Could you check a few things on this model? Use its own coordinates, in mm. Face numbers are marked on the shaded views. A direction names the side the tool comes from. Give positions to 0.01 mm unless a question says otherwise; leave off trailing zeros. Write each loop counter-clockwise with the first axis right and the second up, starting at its lowest first coordinate (ties: lowest second). Pieces come first, ordered by that corner, then holes. Notation, with made-up numbers: (-29.75, -30.5) - (-17.75, -30.5) arc R13 cw to (-17.75, -16.5) - close; hole circle Ø5 at (-21, -9). An arc over 180 degrees is marked (long way). Write item = value, one per line.
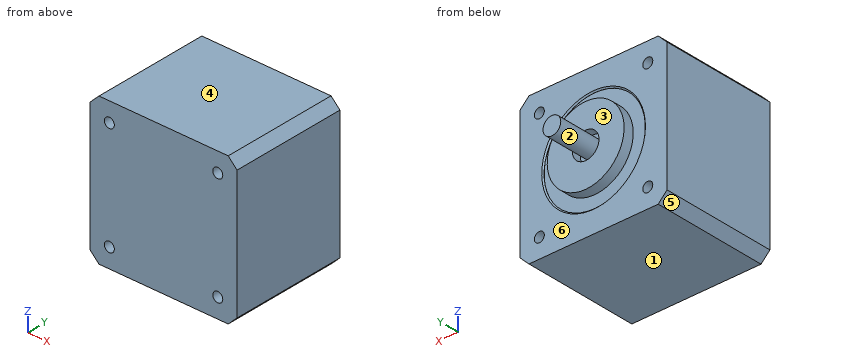
from build123d import *

# Parameters (mm, degrees)
SKETCH1_W           = 42.037
SKETCH1_H           = 42.037
BOSS_EXTRUDE1_DEPTH = 33.02
CHAMFER1_SIZE       = 2.54
SKETCH2_R           = 10.9982
SKETCH2_R_2         = 3.81
BOSS_EXTRUDE2_DEPTH = 2.54
CUT_EXTRUDE1_START  = -0.381
SKETCH3_R           = 14.478
SKETCH3_R_2         = 10.9982
CUT_EXTRUDE1_DEPTH  = 0.381
CHAMFER2_SIZE       = 0.3556
SKETCH4_R           = 2.54
BOSS_EXTRUDE3_DEPTH = 13.3858
SKETCH5_R           = 1.4224
CUT_EXTRUDE2_DEPTH  = 45.428313996


with BuildPart() as part:
    # Sketch1 → Boss-Extrude1 (new body)
    with BuildSketch(Plane(origin=(0, 0, 0), x_dir=(1, 0, 0), z_dir=(0, 1, 0))):
        Rectangle(SKETCH1_W, SKETCH1_H)
    extrude(amount=BOSS_EXTRUDE1_DEPTH)

    # Chamfer1
    chamfer1_edges = [part.edges().sort_by_distance(p)[0] for p in [
        (21.0185, 16.51, 21.0185),
        (-21.0185, 16.51, 21.0185),
        (-21.0185, 16.51, -21.0185),
        (21.0185, 16.51, -21.0185),
    ]]
    chamfer(chamfer1_edges, length=CHAMFER1_SIZE)

    # Sketch2 → Boss-Extrude2 (add)
    with BuildSketch(Plane(origin=(0, 33.02, 0), x_dir=(1, 0, 0), z_dir=(0, 1, 0))):
        with Locations(Location((0, 0, 0), (0, 0, 90))):
            Circle(SKETCH2_R)
        with Locations(Location((0, 0, 0), (0, 0, 270))):
            Circle(SKETCH2_R_2, mode=Mode.SUBTRACT)
    extrude(amount=BOSS_EXTRUDE2_DEPTH)

    # Sketch3 → Cut-Extrude1 (cut)
    with BuildSketch(Plane(origin=(0, 33.02, 0), x_dir=(1, 0, 0), z_dir=(0, 1, 0)).offset(CUT_EXTRUDE1_START)):
        with Locations(Location((0, 0, 0), (0, 0, 270))):
            Circle(SKETCH3_R)
        with Locations(Location((0, 0, 0), (0, 0, 270))):
            Circle(SKETCH3_R_2, mode=Mode.SUBTRACT)
    extrude(amount=CUT_EXTRUDE1_DEPTH, mode=Mode.SUBTRACT)

    # Chamfer2
    chamfer2_edges = [part.edges().sort_by_distance(p)[0] for p in [
        (0, 33.02, -14.478),
    ]]
    chamfer(chamfer2_edges, length=CHAMFER2_SIZE)

    # Sketch4 → Boss-Extrude3 (add)
    with BuildSketch(Plane(origin=(0, 33.02, 0), x_dir=(1, 0, 0), z_dir=(0, 1, 0))):
        with Locations(Location((0, 0, 0), (0, 0, 90))):
            Circle(SKETCH4_R)
    extrude(amount=BOSS_EXTRUDE3_DEPTH)

    # Sketch5 → Cut-Extrude2 (cut, through all)
    with BuildSketch(Plane(origin=(0, 33.02, 0), x_dir=(1, 0, 0), z_dir=(0, 1, 0))):
        with Locations(Location((-15.5067, 15.5067, 0), (0, 0, 270))):
            Circle(SKETCH5_R)
        with Locations(Location((15.5067, 15.5067, 0), (0, 0, 270))):
            Circle(SKETCH5_R)
        with Locations(Location((-15.5067, -15.5067, 0), (0, 0, 270))):
            Circle(SKETCH5_R)
        with Locations(Location((15.5067, -15.5067, 0), (0, 0, 270))):
            Circle(SKETCH5_R)
    extrude(amount=-CUT_EXTRUDE2_DEPTH, mode=Mode.SUBTRACT)


solid = part.part
1. Which directions (+Z, -Z, +X, -X, +Y, -Y) give clear straight access to the entire face, cutting with the end or side of a thin tool? Please do the marked faces 5 and 6.
Filled sheet:
face_5 = -Z, -X, +Y, -Y
face_6 = +Y
2. Thinking about a two-plate mould opening in Z: for the marked faces 1, 2, 3 and 4, which applies, pulls with the +Z half, pulls with the -Z half, needs draft (parallel to the pull), parting line crosses it, or undercut?
Filled sheet:
face_1 = pulls with the -Z half
face_2 = undercut
face_3 = needs draft
face_4 = pulls with the +Z half
3. If we section it at B-B, the plane y = 19: Please give me the cut outline in (x, z), and give its area (3 significant figures).
Filled sheet:
outline = (-21.02, -18.48) - (-18.48, -21.02) - (18.48, -21.02) - (21.02, -18.48) - (21.02, 18.48) - (18.48, 21.02) - (-18.48, 21.02) - (-21.02, 18.48) - close; hole circle Ø2.84 at (-15.51, -15.51); hole circle Ø2.84 at (-15.51, 15.51); hole circle Ø2.84 at (15.51, -15.51); hole circle Ø2.84 at (15.51, 15.51)
area = 1,730 mm2
4. For pin 1 (1.7 mm diameter, centred on x = 15.51, z = -15.51, fed in from -Y); pin 2 (1.5 mm diameter, centred on y = 34, z = 0, fed in from -X); pin 3 (3.5 mm diameter, centred on x = -15.51, z = 15.51, fed in from +Y); pin 4 (8.5 mm diameter, centred on x = -4.5, z = 5.5, fed in from +Y), each with a flat end and sliding along its axis, tell me the tip position at first contact or that it passes through.
Filled sheet:
pin_1 = through
pin_2 = -11
pin_3 = 33.02
pin_4 = 35.56
5. I need wall thicknesses on line 1 (Z direction, x = -16.5, y = 11.5); line 2 (X direction, y = 15, z = -15); line 3 (Y direction, x = -15.5, z = 0). Which ranges of each line are inside material? Lowest first, please.
Filled sheet:
line_1 = -21.02 to -16.52, -14.49 to 14.49, 16.52 to 21.02
line_2 = -21.02 to -16.84, -14.18 to 14.18, 16.84 to 21.02
line_3 = 0 to 33.02
